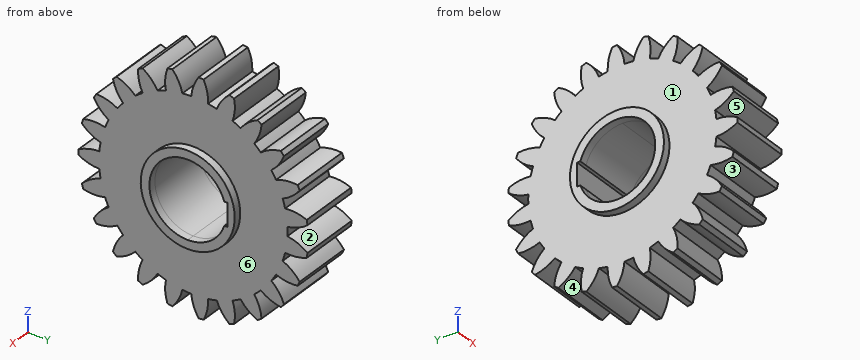
from build123d import *
from build123d.topology import SkipClean

# Parameters (mm, degrees)
BASPROSKE_W         = 4
BASPROSKE_H         = 7.5
TOOTHCUT_DEPTH      = 12.335784049
TEETHCUTS_COUNT     = 23
TEETHCUTS_ANGLE     = 344.347826087
BORSKE_R            = 2.5
BORE_DEPTH          = 50.0000508
EXTRUDE1_DEPTH      = 0.5
EXTRUDE1_DEPTH_BACK = 4.5
SKETCH1_R           = 3.065937152
SKETCH1_R_2         = 2.5
SKETCH2_W           = 1.5
SKETCH2_H           = 2.6
CUT_EXTRUDE1_DEPTH  = 5.5


with BuildPart() as part:
    # BasProSke → Base-Revolve (revolve)
    with BuildSketch(Plane(origin=(0, 0, 0), x_dir=(1, 0, 0), z_dir=(0, 1, 0)), mode=Mode.PRIVATE) as base_revolve_sk:
        with Locations((2, 3.75)):
            Rectangle(BASPROSKE_W, BASPROSKE_H)
    revolve(base_revolve_sk.sketch.rotate(Axis((-10, 0, 0), (1, 0, 0)), 180), axis=Axis((-10, 0, 0), (1, 0, 0)))

    # TooCutSke → ToothCut (cut, through all)
    with BuildSketch(Plane(origin=(0, 0, 0), x_dir=(0, 0, -1), z_dir=(1, 0, 0))):
        with BuildLine():
            ThreePointArc((0.292498096, 6.142039227), (0, 6.149), (-0.292498096, 6.142039227))
            ThreePointArc((-0.292498096, 6.142039227), (-0.495998432, 6.847302274), (-0.878204189, 7.473981707))
            ThreePointArc((-0.878204189, 7.473981707), (0, 7.5254), (0.878204189, 7.473981707))
            ThreePointArc((0.878204189, 7.473981707), (0.495998432, 6.847302274), (0.292498096, 6.142039227))
        make_face()
    toothcut = extrude(amount=TOOTHCUT_DEPTH, mode=Mode.SUBTRACT)

    # TeethCuts: ToothCut ×23 about axis
    teethcuts_axis = Axis((-10, 0, 0), (1, 0, 0))
    for i in range(1, TEETHCUTS_COUNT):
        add(toothcut.rotate(teethcuts_axis, i * TEETHCUTS_ANGLE / (TEETHCUTS_COUNT - 1)), mode=Mode.SUBTRACT)

    # BorSke → Bore (cut, symmetric)
    with BuildSketch(Plane(origin=(0, 0, 0), x_dir=(0, 0, -1), z_dir=(1, 0, 0))):
        with Locations(Location((0, 0, 0), (0, 0, 180))):
            Circle(BORSKE_R)
    extrude(amount=BORE_DEPTH, both=True, mode=Mode.SUBTRACT)

    # Sketch1 → Extrude1 (add, two sides: drawn at the far end of the back side and taken through both)
    with SkipClean():  # the faces are left unmerged after this step: merging them gives an invalid solid
        with BuildSketch(Plane(origin=(4, 0, 0), x_dir=(0, 0, -1), z_dir=(1, 0, 0)).offset(-EXTRUDE1_DEPTH_BACK)):
            Circle(SKETCH1_R)
            Circle(SKETCH1_R_2, mode=Mode.SUBTRACT)
        extrude(amount=EXTRUDE1_DEPTH + EXTRUDE1_DEPTH_BACK)
    add(part.part.scale(1), mode=Mode.REPLACE)  # the faces are merged on a copy

    # Sketch2 → Cut-Extrude1 (cut)
    with SkipClean():  # the faces are left unmerged after this step: merging them gives an invalid solid
        with BuildSketch(Plane(origin=(4.5, 0, 0), x_dir=(0, 0, -1), z_dir=(1, 0, 0))):
            with Locations((0, 1.3)):
                Rectangle(SKETCH2_W, SKETCH2_H)
        extrude(amount=-CUT_EXTRUDE1_DEPTH, mode=Mode.SUBTRACT)


solid = part.part
The model under review builds one solid part; all positions refer to its coordinate system, in mm. Face numbers are marked on the shaded views. A direction names the side the tool comes from. Coordinates: 2 decimals unless noted, no trailing zeros. Loops run counter-clockwise (first coordinate to the right, second up) from the corner with the lowest first, then second, coordinate; pieces in that order, holes last. Notation, with made-up numbers: M 36.25,-9 L 51.25,-9 A14 ccw 51.25,4 Z; hole C -33,26 d5. An arc over 180 degrees is marked long. Put each result on its own line as item: value. Start each with the question number.
Q1. Clearance check with flat-ended pins moving along their axes: pin 1 (1.5 mm diameter, centred on y = -5, z = -4.5, fed in from -X); pin 2 (2 mm diameter, centred on x = 1.5, z = 4.5, fed in from -Y); pin 3 (1.5 mm diameter, centred on y = -0.5, z = 4, fed in from +X). State where each tip first meets the part, or that it passes through.
Q2. The part is to be moulded in two halves that separate along Y. For the marked faces 1, 2 and 3, say which applies: +Y half, -Y half, draft (parallel to the pull), parting line (faces both ways), or undercut.
Q3. Wall thickness on line 1 (Z direction, x = 4.2, y = 0); line 2 (Y direction, x = 4.15, z = 0); line 3 (X direction, y = 3.25, z = 5): over which ranges is each line inside the solid? List them lowest first.
Q4. Add section A-A (x = -0.2). Write out the cut boundary in (y, z), and give its area (3 significant figures).
Q5. For the marked faces 4, 5 and 6, list the 3-axis set-ups (+Z, -Z, +X, -X, +Y, -Y) from which the entire face can be reached by the end or side of a thin tool; tool diameter is ignored.
Answers:
1. pin 1: stops at x = 0
1. pin 2: stops at y = -6.49
1. pin 3: stops at x = 4
2. face 1: draft
2. face 2: +Y half
2. face 3: undercut
3. line 1: z = -3.07 to -2.5, 2.5 to 3.07
3. line 2: y = -3.07 to -2.5, 2.6 to 3.07
3. line 3: x = 0 to 4
4. outline: C 0,0 d6.13; hole M 2.38,-0.75 L 2.6,-0.75 L 2.6,0.75 L 2.38,0.75 A2.5 ccw long Z
4. area: 9.69 mm^2
5. face 4: -Z, +X, -X
5. face 5: +X, -X, -Y
5. face 6: +X
